from build123d import *

# Parameters (mm, degrees)
F0_W      = 79.5655027032
F0_H      = 36.2267494202
F1_DEPTH  = 12.7
F2_DEPTH  = 12.7
F3_R      = 11.1269376105
F4_DEPTH  = 177.8
F7_DEPTH  = 50.8
F8_DEPTH  = 50.8
F11_DEPTH = 6.35
F12_SIZE  = 5.08
F13_DEPTH = 6.35
F14_SIZE  = 5.08
F15_R     = 7.62
F16_R     = 7.62


with BuildPart() as f1:
    # F0 (on Top) → F1 (new body)
    with BuildSketch(Plane.XY):
        with Locations((-0.5556233227, -0.4444997758)):
            Rectangle(F0_W, F0_H)
    extrude(amount=F1_DEPTH)

    # F2 (add): a face of the model
    f2_faces = [f1.faces().sort_by_distance(p)[0] for p in [
        (-0.5556233227, -0.4444997758, 0),
    ]]
    extrude(f2_faces, amount=F2_DEPTH)

    # F3 (on face) → F4 (join)
    with BuildSketch(Plane(origin=(0, 0, -12.7), x_dir=(1, 0, 0), z_dir=(0, 0, -1))):
        Circle(F3_R)
    extrude(amount=F4_DEPTH)

    # F7 (add): a face of the model
    f7_faces = [f1.faces().sort_by_distance(p)[0] for p in [
        (-40.3383746743, -0.4444997758, 0),
    ]]
    extrude(f7_faces, amount=F7_DEPTH)

    # F8 (add): a face of the model
    f8_faces = [f1.faces().sort_by_distance(p)[0] for p in [
        (39.2271280289, -0.4444997758, 0),
    ]]
    extrude(f8_faces, amount=F8_DEPTH)

    # F9 (on face) → F11 (join)
    with BuildSketch(Plane.XZ.offset(18.5578744859)):
        Polygon((11.0919512808, -12.7), (-0.5556233227, 12.7), (-12.2015299276, -12.7), align=None)
        Polygon((46.031339094, 12.7), (22.7378578857, 12.7), (34.3854324892, -12.7), align=None)
        Polygon((69.3248221651, 12.7), (57.6780801639, -12.7), (80.9723967686, -12.7), align=None)
        Polygon((-35.4950129986, -12.7), (-23.8482709974, 12.7), (-47.1425876021, 12.7), align=None)
        Polygon((-82.083646208, -12.7), (-58.7893296033, -12.7), (-70.4369042069, 12.7), align=None)
    extrude(amount=F11_DEPTH)

    # F12
    f12_edges = [f1.edges().sort_by_distance(p)[0] for p in [
        (-70.436488, -24.907874, -12.7),
        (-64.613117, -24.907874, 0),
        (-76.260275, -24.907874, 0),
        (-41.3188, -24.907874, 0),
        (-29.671642, -24.907874, 0),
        (-35.495429, -24.907874, 12.7),
        (5.268164, -24.907874, 0),
        (-6.378577, -24.907874, 0),
        (-0.554789, -24.907874, -12.7),
        (34.384598, -24.907874, 12.7),
        (28.561645, -24.907874, 0),
        (40.208386, -24.907874, 0),
        (75.148609, -24.907874, 0),
        (63.501451, -24.907874, 0),
        (69.325238, -24.907874, -12.7),
    ]]
    chamfer(f12_edges, length=F12_SIZE)

    # F10 (on face) → F13 (join)
    with BuildSketch(Plane(origin=(0, 17.6688749343, 0), x_dir=(-1, 0, 0), z_dir=(0, 1, 0))):
        Polygon((12.1067352593, -12.7), (0.5556233227, 12.7), (-10.8906552196, -12.7), align=None)
        Polygon((47.2631566226, 12.7), (23.6892774701, 12.7), (35.5443507433, -12.7), align=None)
        Polygon((70.291981101, 12.7), (58.8457025588, -12.7), (81.8430930376, -12.7), align=None)
        Polygon((-33.8880456984, -12.7), (-22.4417671561, 12.7), (-45.439157635, 12.7), align=None)
        Polygon((-79.8828266561, -12.7), (-56.8854361773, -12.7), (-68.4365481138, 12.7), align=None)
    extrude(amount=F13_DEPTH)

    # F14
    f14_edges = [f1.edges().sort_by_distance(p)[0] for p in [
        (68.384131, 24.018875, -12.7),
        (62.660992, 24.018875, 0),
        (74.159687, 24.018875, 0),
        (28.164906, 24.018875, 0),
        (33.940462, 24.018875, 12.7),
        (39.663602, 24.018875, 0),
        (-0.60804, 24.018875, -12.7),
        (-6.331179, 24.018875, 0),
        (5.167516, 24.018875, 0),
        (-35.476217, 24.018875, 12.7),
        (-29.616814, 24.018875, 0),
        (-41.403754, 24.018875, 0),
        (-76.067537, 24.018875, 0),
        (-64.568842, 24.018875, 0),
        (-70.344398, 24.018875, -12.7),
    ]]
    chamfer(f14_edges, length=F14_SIZE)

    # F15
    f15_edges = [f1.edges().sort_by_distance(p)[0] for p in [
        (90.027128, -0.4445, 12.7),
        (90.027128, 17.668875, 0),
        (90.027128, -0.4445, -12.7),
        (90.027128, -18.557874, 0),
    ]]
    fillet(f15_edges, radius=F15_R)

    # F16
    f16_edges = [f1.edges().sort_by_distance(p)[0] for p in [
        (-91.138375, 17.668875, 0),
        (-91.138375, -0.4445, 12.7),
        (-91.138375, -18.557874, 0),
        (-91.138375, -0.4445, -12.7),
    ]]
    fillet(f16_edges, radius=F16_R)


solid = f1.part
Source: CAD feature listing. Evaluate the final solid. Frame: model axes, mm. A direction names the side the tool comes from. Coordinates: 2 decimals unless noted, no trailing zeros. Order: outer loops, then holes, each group sorted by start corner. A loop starts at its lowest first (then second) coordinate and runs counter-clockwise, first axis right, second up. Notation, with made-up numbers: M 11.5,16 L 65.5,16 A13 ccw 65.5,23 Z; hole C -13.75,81 d5. An arc over 180 degrees is marked long. Write each question's results on one line, items separated by ' | '. Start each with the question number.
Item 1: Cut plane B-B (x = -62). Return loops of the section in (y, z).
Item 2: Cut plane A-A (y = 0). Return loops of the section in (x, z), and give its area (3 significant figures).
Item 3: First-contact query: pin 1 Ø7.5 at (x, z) = (52.5, -1.5) entering from -Y; pin 2 Ø1 at (x, y) = (-52, 15.5) entering from -Z; pin 3 Ø7.5 at (x, z) = (-60.5, 4.5) entering from +Y. Flat tips, straight axial feed; report the tip coordinate or a pass-through.
Item 4: Cut plane D-D (x = 54). Return loops of the section in (y, z).
Item 5: Draft query along X for faces 4 (the face through (-41.32, 18.29, -0.18)), 5 (the face through (-1, 24.019, -4)), 6 (the face through (86.85, -17.13, 0.18)). Return one class per face: pulls with the +X half, pulls with the -X half, needs draft (parallel to the pull), parting line crosses it, or undercut.
Item 6: Set-up query: faces 1 (the face through (77, 17.669, 3)), 2 (the face through (-64.53, -19.18, -0.18)), 3 (the face through (-66.48, 20.95, -0.65)). Return all of +Z, -Z, +X, -X, +Y, -Y with unobstructed straight access to the full face (end or side cutting, diameter ignored); none if empty.
Item 7: Line query: probe 1 along X at (y, z) = (1, -118.5); probe 2 along Z at (x, y) = (-57.5, -14); probe 3 along Y at (x, z) = (26.5, -10.5). Output: solid intervals per line, ascending.
Item 8: Cut plane C-C (z = -94). Return loops of the section in (x, y).
Checked values:
1) outline: M -21.89,-10.64 L -19.83,-12.7 L 18.94,-12.7 L 20.98,-10.66 L 18.94,-5.7 L 17.67,-5.7 L 17.67,12.7 L -18.56,12.7 L -18.56,-5.7 L -19.83,-5.7 Z
2) outline: M -91.14,-5.08 A7.62 ccw -83.52,-12.7 L -11.13,-12.7 L -11.13,-190.5 L 11.13,-190.5 L 11.13,-12.7 L 82.41,-12.7 A7.62 ccw 90.03,-5.08 L 90.03,5.08 A7.62 ccw 82.41,12.7 L -83.52,12.7 A7.62 ccw -91.14,5.08 Z | area: 8,510 mm2
3) pin 1: stops at y = -18.56 | pin 2: stops at z = -12.7 | pin 3: stops at y = 17.67
4) outline: M -18.56,-12.7 L 17.67,-12.7 L 17.67,12.7 L -18.56,12.7 Z
5) face 4: undercut | face 5: needs draft | face 6: pulls with the +X half
6) face 1: +Z, +X, +Y | face 2: +Z, -Y | face 3: +Z, +Y
7) probe 1: x = -11.08 to 11.08 | probe 2: z = -12.7 to 12.7 | probe 3: y = -18.56 to 17.67
8) outline: C 0,0 d22.25
